Read the model definition and answer for the solid it produces. Units are mm, in the model's axes. Face numbers are marked on the shaded views. A direction names the side the tool comes from. Give positions to 0.01 mm unless a question says otherwise; leave off trailing zeros. Loops run counter-clockwise (first coordinate to the right, second up) from the corner with the lowest first, then second, coordinate; pieces in that order, holes last. Notation, with made-up numbers: (-3.75, 77.5) -> (52.25, 77.5) arc R14 ccw to (52.25, 102.5) -> close; hole circle Ø3 at (-18, 79.5). An arc over 180 degrees is marked (long way). Write each question's results on one line, items separated by ' | '. Start each with the question number.
Item 1: Section A-A on z = 11.5 is taken. Write down the section's boundary in (x, y), and give its area (3 significant figures).
Item 2: Section B-B on y = -60 is taken. Write down the section's boundary in (x, z), and give its area (3 significant figures).
Item 3: Determine the mould class of the marked faces 3, 4, 5 and 6 for opening direction X: +X half, -X half, draft (parallel to the pull), parting line (faces both ways), or undercut.
Item 4: Which of the six approach directions +Z, -Z, +X, -X, +Y, -Y give full straight-line access (tool end or side, diameter ignored) to the marked faces 1 and 2?
Item 5: Find the intervals of material crossed by line 1 (X direction, y = -24.5, z = 15.75); line 2 (Y direction, x = 63, z = 8); line 3 (Z direction, x = 92.5, y = -62), in increasing order.
Item 6: Section C-C on x = 59 is taken. Write down the section's boundary in (y, z), and give its area (3 significant figures).
```python
from build123d import *

# Parameters (mm, degrees)
F0_W     = 153.124735
F0_H     = 86.703286
F1_DEPTH = 25.4
F2_R     = 5.08
F3_T     = -2.54


with BuildPart() as f1:
    # F0 (on Top) → F1 (new body)
    with BuildSketch(Plane.XY):
        with Locations((76.562367, -43.351643)):
            Rectangle(F0_W, F0_H)
    extrude(amount=F1_DEPTH)

    # F2
    f2_edges = [f1.edges().sort_by_distance(p)[0] for p in [
        (0, -43.351643, 25.4),
        (76.562367, -86.703286, 25.4),
        (76.562367, 0, 25.4),
        (153.124735, -43.351643, 25.4),
    ]]
    fillet(f2_edges, radius=F2_R)

    # F3
    f3_openings = [f1.faces().sort_by_distance(p)[0] for p in [
        (76.562367, -43.351643, 0),
    ]]
    offset(amount=F3_T, openings=f3_openings)


solid = f1.part
```
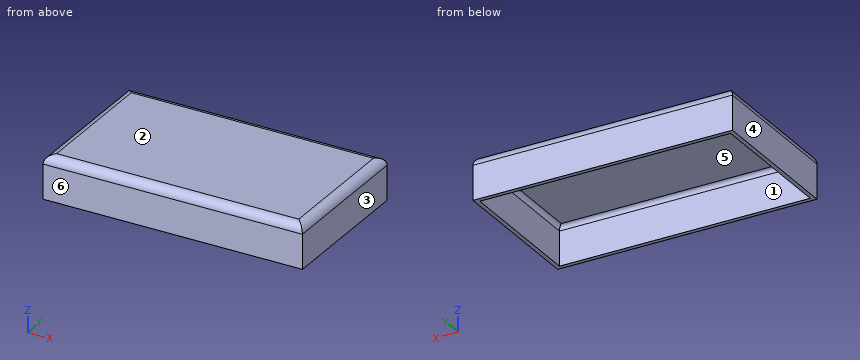
Findings:
1) outline: (0, -86.7) -> (153.12, -86.7) -> (153.12, 0) -> (0, 0) -> close; hole (2.54, -84.16) -> (150.58, -84.16) -> (150.58, -2.54) -> (2.54, -2.54) -> close | area: 1,190 mm2
2) outline: (0, 0) -> (2.54, 0) -> (2.54, 20.32) arc R2.54 cw to (5.08, 22.86) -> (148.04, 22.86) arc R2.54 cw to (150.58, 20.32) -> (150.58, 0) -> (153.12, 0) -> (153.12, 20.32) arc R5.08 ccw to (148.04, 25.4) -> (5.08, 25.4) arc R5.08 ccw to (0, 20.32) -> close | area: 497 mm2
3) face 3: +X half | face 4: -X half | face 5: undercut | face 6: draft
4) face 1: -Z | face 2: +Z, +X, -X, +Y, -Y
5) line 1: 0 to 2.54, 150.58 to 153.12 | line 2: -86.7 to -84.16, -2.54 to 0 | line 3: 22.86 to 25.4
6) outline: (-86.7, 0) -> (-84.16, 0) -> (-84.16, 20.32) arc R2.54 cw to (-81.62, 22.86) -> (-5.08, 22.86) arc R2.54 cw to (-2.54, 20.32) -> (-2.54, 0) -> (0, 0) -> (0, 20.32) arc R5.08 ccw to (-5.08, 25.4) -> (-81.62, 25.4) arc R5.08 ccw to (-86.7, 20.32) -> close | area: 328 mm2
